Geometry check sheet. Reference: drawing and pictorial views, mm from the part's lowest x, y, z. A direction names the side the tool comes from. Round coordinates to 2 decimals unless told otherwise and drop trailing zeros. Order: outer loops, then holes, each group sorted by start corner. A loop starts at its lowest first (then second) coordinate and runs counter-clockwise, first axis right, second up.
(1) Sectioned sample at A-A (z = 1.25). Record the boundary of the cut face in (x, y), plus the area to 3 significant figures.
(2) Material ranges on line 1 along Y through (x, z) = (3.25, 1) (1 decimal); line 2 along X through (y, z) = (5.25, 7.75); line 3 along Y through (x, z) = (5.75, 7.5) (1 decimal), recorded low to high.
(3) Release check for a two-part mould opening along X. For the marked faces 1, 2 and 3 record: +X half, -X half, draft (parallel to the pull), parting line (faces both ways), or undercut.
(4) Sectioned sample at C-C (z = 10.5). Record the boundary of the cut face in (x, y).
(5) Go/stop test with flat-tipped pins: pin 1 (1 mm diameter, centred on y = 3, z = 11, fed in from +X); pin 2 (3 mm diameter, centred on x = 4.5, z = 11, fed in from -Y); pin 3 (1 mm diameter, centred on y = 4, z = 10, fed in from +X). Record where each tip stops, or that it passes through.
(6) Set-up check for the marked faces 4 and 5: record each of +Z, -Z, +X, -X, +Y, -Y from which the full face is reachable in a straight line by a thin tool's end or side.
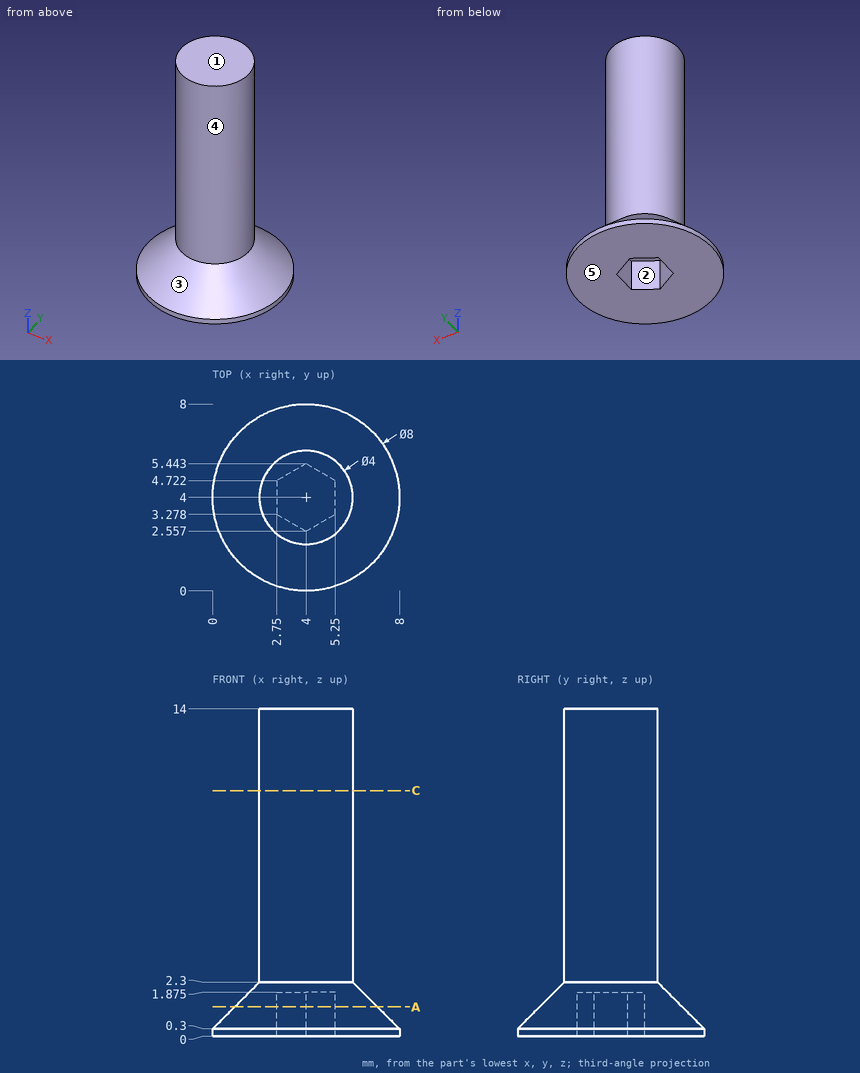
Answer below:
1. outline: circle Ø6.1 at (4, 4); hole (2.75, 3.28) - (4, 2.56) - (5.25, 3.28) - (5.25, 4.72) - (4, 5.44) - (2.75, 4.72) - close
1. area: 23.8 mm2
2. line 1: y = 0.8 to 3, 5 to 7.2
2. line 2: x = 2.44 to 5.56
2. line 3: y = 3 to 5
3. face 1: draft
3. face 2: undercut
3. face 3: parting line
4. outline: circle Ø4 at (4, 4)
5. pin 1: stops at x = 5.94
5. pin 2: stops at y = 2
5. pin 3: stops at x = 6
6. face 4: +Z
6. face 5: -Z, +X, -X, +Y, -Y
